```python
from build123d import *

# Parameters (mm, degrees)
F2_SIZE = 5


with BuildPart() as f1:
    # F0 (on Front) → F1 (revolve)
    with BuildSketch(Plane.XZ):
        Polygon((20, 0), (0, 0), (0, -35), (90, -35), (90, -10), (80, 0), (30, 0), (30, -17.5), (20, -14.8205080757), align=None)
    revolve(axis=Axis((44.4514416158, 0, -45), (1, 0, 0)))

    # F2
    f2_edges = [f1.edges().sort_by_distance(p)[0] for p in [
        (0, 0, -90),
        (20, 0, -90),
        (30, 0, -90),
        (0, 0, -55),
        (90, 0, -55),
    ]]
    chamfer(f2_edges, length=F2_SIZE)


solid = f1.part
```
The listing builds one solid part. Answer for the finished solid, in the listing's coordinates (mm). A direction names the side the tool comes from. Round coordinates to 2 decimals unless told otherwise and drop trailing zeros. Loops run counter-clockwise (first coordinate to the right, second up) from the corner with the lowest first, then second, coordinate; pieces in that order, holes last. Notation, with made-up numbers: (52, -22) - (66, -22) arc R26 cw to (66, 17) - close; hole circle Ø7 at (-39.5, 35). An arc over 180 degrees is marked (long way). Return JSON: item names as keys, results as strings. Group by question number.
1. The mould has two halves that part along Z. Classify faces 1 (the conical face through (89.374, -1.566, -80.591)), 2 (the flat face through (90, 7, -60)), 3 (the conical face through (4.76, -0.45, -55.23)), 4 (the cylindrical face through (46, 0, -55)): pulls with the +Z half, pulls with the -Z half, needs draft (parallel to the pull), parting line crosses it, or undercut.
2. Each of these flat-tipped pins is pushed along its axis until it touches: P1, Ø4, axis at x = 23.5, y = -5.5, coming from the +Z side; P2, Ø1.5, axis at x = 17.5, y = -1, coming from the -Z side; P3, Ø1.5, axis at x = 52.5, y = 28, coming from the +Z side. Where does it stop, or does it pass through?
3. The part is cut by section D-D on x = 27. Determine the outline of the cut face in (y, z), then the cut area to 3 significant figures.
4. Which of the six approach directions +Z, -Z, +X, -X, +Y, -Y give full straight-line access (tool end or side, diameter ignored) to faces 5 (the cylindrical face through (9.93, -1.979, -89.956)), 6 (the flat face through (20, -30, -51))?
5. The part is cut by section A-A on z = -45. Determine the outline of the cut face in (x, y).
6. The part is cut by section C-C on x = 63.5. Determine the outline of the cut face in (y, z).
7. Consider probe 1 along Y at (x, z) = (37.5, -45); probe 2 along Z at (x, y) = (60, 0); probe 3 along X at (y, z) = (27, -66). Determine where each line is inside the solid, lowest interval first.
8. The part is cut by section B-B on y = 0. Determine the outline of the cut face in (x, z).
Resolved:
{
 "1": {"face 1": "parting line crosses it", "face 2": "needs draft", "face 3": "undercut", "face 4": "undercut"},
 "2": {"P1": "stops at z = -15.64", "P2": "stops at z = -88.24", "P3": "stops at z = -9.19"},
 "3": {"outline": "circle Ø56.61 at (0, -45); hole circle Ø20 at (0, -45)", "area": "2,200 mm²"},
 "4": {"face 5": "+X, -X", "face 6": "none"},
 "5": {"outline": "(0, -40) - (5, -45) - (15, -45) - (20, -40) - (20, -30.18) - (30, -27.5) - (30, -40) - (35, -45) - (80, -45) - (90, -35) - (90, -15) - (85, -10) - (5, -10) - (0, -15) - close; (0, 15) - (5, 10) - (85, 10) - (90, 15) - (90, 35) - (80, 45) - (35, 45) - (30, 40) - (30, 27.5) - (20, 30.18) - (20, 40) - (15, 45) - (5, 45) - (0, 40) - close"},
 "6": {"outline": "circle Ø90 at (0, -45); hole circle Ø20 at (0, -45)"},
 "7": {"probe 1": "y = -45 to -10, 10 to 45", "probe 2": "z = -90 to -55, -35 to 0", "probe 3": "x = 0 to 20, 30 to 90"},
 "8": {"outline": "(0, -85) - (5, -90) - (15, -90) - (20, -85) - (20, -75.18) - (30, -72.5) - (30, -85) - (35, -90) - (80, -90) - (90, -80) - (90, -60) - (85, -55) - (5, -55) - (0, -60) - close; (0, -30) - (5, -35) - (85, -35) - (90, -30) - (90, -10) - (80, 0) - (35, 0) - (30, -5) - (30, -17.5) - (20, -14.82) - (20, -5) - (15, 0) - (5, 0) - (0, -5) - close"}
}
